```python
from build123d import *

# Parameters (mm, degrees)
BOSS_EXTRUDE1_DEPTH     = 63.5
SKETCH2_R               = 14.2875
CUT_EXTRUDE1_DEPTH      = 100.9999
M4_CLEARANCE_HOLE1_D    = 4.5
F_1_4_CLEARANCE_HOLE1_D = 6.7564


with BuildPart() as part:
    # Sketch1 → Boss-Extrude1 (new body)
    with BuildSketch(Plane(origin=(0, 0, 0), x_dir=(0, 0, -1), z_dir=(1, 0, 0))):
        Polygon((0, 0), (0, 3.175), (48.26, 3.175), (48.26, 15.875), (54.61, 15.875), (54.61, 3.175), (76.2, 3.175), (76.2, 0), align=None)
    extrude(amount=BOSS_EXTRUDE1_DEPTH)

    # Sketch2 → Cut-Extrude1 (cut, through all)
    with BuildSketch(Plane(origin=(0, 3.175, 0), x_dir=(1, 0, 0), z_dir=(0, 1, 0))):
        with Locations(Location((31.75, 33.685553713, 0), (0, 0, 270))):
            Circle(SKETCH2_R)
    extrude(amount=-CUT_EXTRUDE1_DEPTH, mode=Mode.SUBTRACT)

    # M4 Clearance Hole1 (through all)
    with Locations(Plane(origin=(0, 0, 0), x_dir=(-1, 0, 0), z_dir=(0, -1, 0))):
        with Locations((-31.75, 12.185553713), (-50.369546181, 44.435553713), (-13.130453819, 44.435553713)):
            Hole(M4_CLEARANCE_HOLE1_D / 2)

    # 1/4 Clearance Hole1 (through all)
    with Locations(Plane.XY.offset(-48.26)):
        with Locations((41.91, 8.9662), (21.59, 8.9662)):
            Hole(F_1_4_CLEARANCE_HOLE1_D / 2)


solid = part.part
```
Read the model definition and answer for the solid it produces. Units are mm, in the model's axes. A direction names the side the tool comes from. Round coordinates to 2 decimals unless told otherwise and drop trailing zeros. Write each loop counter-clockwise with the first axis right and the second up, starting at its lowest first coordinate (ties: lowest second). Pieces come first, ordered by that corner, then holes. Notation, with made-up numbers: (7, 77.25) -> (51, 77.25) arc R28 cw to (51, 109.25) -> close; hole circle Ø9 at (-8.5, 62.25). An arc over 180 degrees is marked (long way). Answer in a Markdown table with one row per item. Add a question column.
1) Determine the mould class of faces 1 (the face through (45.285, 9.115, -51.479)), 2 (the face through (24, 0, -47)), 3 (the face through (63.5, 3, -41)) for opening direction Y: pulls with the +Y half, pulls with the -Y half, needs draft (parallel to the pull), parting line crosses it, or undercut.
2) Find section B-B, the plane z = -38. Determine the outline of the cut face in (x, y) (1 decimal), and give its area (3 significant figures).
3) Find section C-C, the plane y = 6.75. Determine the outline of the cut face in (x, z).
4) Find section D-D, the plane x = 5.5. Determine the outline of the cut face in (y, z) (3 decimals).
5) Which of the six approach directions +Z, -Z, +X, -X, +Y, -Y give full straight-line access (tool end or side, diameter ignored) to faces 4 (the face through (31, 3.175, -18)), 5 (the face through (31, 3.175, -65)), 6 (the face through (19.075, 1.61, -27.093))?
6) Consider line 1 (Y direction, x = 23.5, z = -60) (3 decimals); line 2 (Z direction, x = 52, y = 14.75). Determine where each line is inside the solid, lowest interval first.
7) Find section A-A, the plane x = 31.75. Determine the outline of the cut face in (y, z) (3 decimals), and give its area (3 significant figures).
8) Given P1, Ø4, axis at x = 41.91, y = 8.97, coming from the -Z side; P2, Ø2, axis at x = 37, z = -10.5, coming from the +Y side (3 decimals); P3, Ø4, axis at x = 56, y = 11, coming from the +Z side, each flat-ended and moving along its own axis, determine where each tip first touches the part or whether it passes through.
Findings below:
| question | item | result |
|---|---|---|
| 1 | face 1 | undercut |
| 1 | face 2 | pulls with the -Y half |
| 1 | face 3 | needs draft |
| 2 | outline | (0, 0) -> (18.1, 0) -> (18.1, 3.2) -> (0, 3.2) -> close; (45.4, 0) -> (63.5, 0) -> (63.5, 3.2) -> (45.4, 3.2) -> close |
| 2 | area | 115 mm² |
| 3 | outline | (0, -54.61) -> (19.04, -54.61) -> (19.04, -48.26) -> (0, -48.26) -> close; (24.14, -54.61) -> (39.36, -54.61) -> (39.36, -48.26) -> (24.14, -48.26) -> close; (44.46, -54.61) -> (63.5, -54.61) -> (63.5, -48.26) -> (44.46, -48.26) -> close |
| 4 | outline | (0, -76.2) -> (3.175, -76.2) -> (3.175, -54.61) -> (15.875, -54.61) -> (15.875, -48.26) -> (3.175, -48.26) -> (3.175, 0) -> (0, 0) -> close |
| 5 | face 4 | +Z, +X, -X, +Y |
| 5 | face 5 | -Z, +X, -X, +Y |
| 5 | face 6 | +Y, -Y |
| 6 | line 1 | 0 to 3.175 |
| 6 | line 2 | -54.61 to -48.26 |
| 7 | outline | (0, -76.2) -> (3.175, -76.2) -> (3.175, -54.61) -> (15.875, -54.61) -> (15.875, -48.26) -> (3.175, -48.26) -> (3.175, -47.973) -> (0, -47.973) -> close; (0, -19.398) -> (3.175, -19.398) -> (3.175, -14.436) -> (0, -14.436) -> close; (0, -9.936) -> (3.175, -9.936) -> (3.175, 0) -> (0, 0) -> close |
| 7 | area | 218 mm² |
| 8 | P1 | through |
| 8 | P2 | y = 3.175 |
| 8 | P3 | z = -48.26 |
